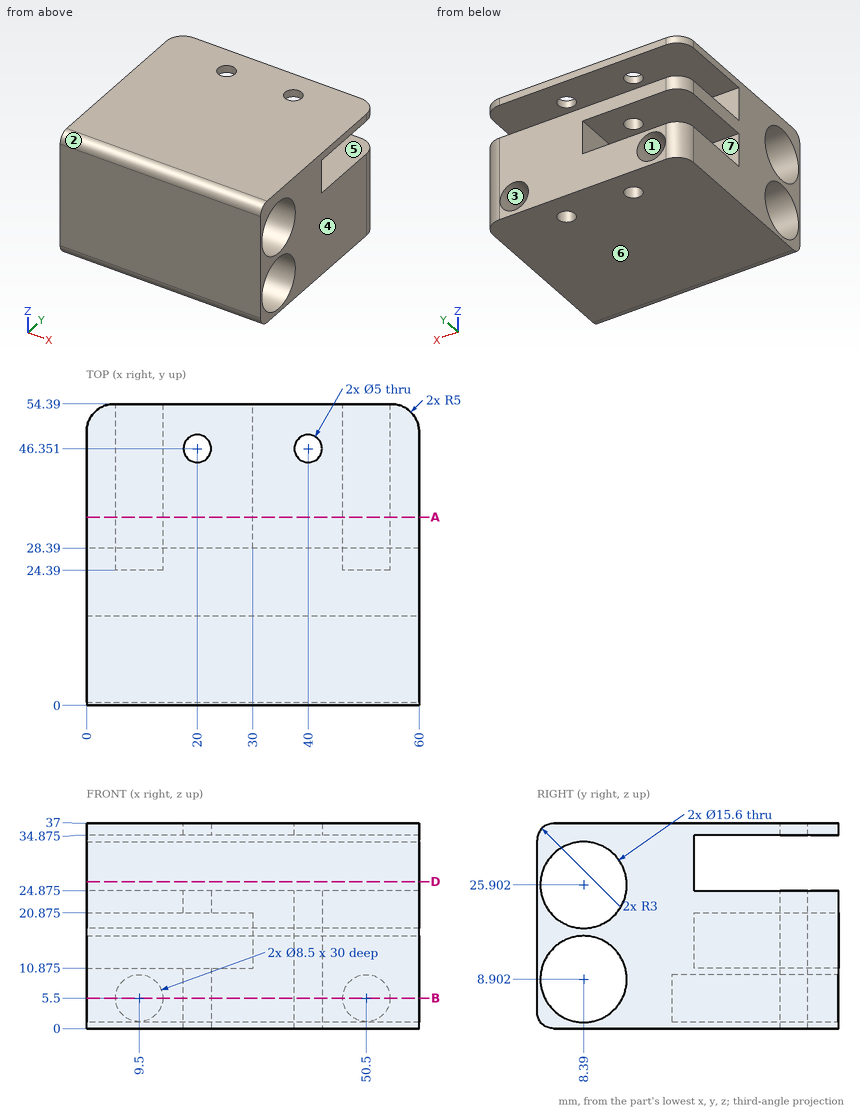
Source: three-view drawing plus pictorial views. Frame: mm from the lowest corner of the part. A direction names the side the tool comes from. Give positions to 0.01 mm unless a question says otherwise; leave off trailing zeros. Order: outer loops, then holes, each group sorted by start corner. A loop starts at its lowest first (then second) coordinate and runs counter-clockwise, first axis right, second up. Notation, with made-up numbers: (-5.75, 69.5) -> (53.25, 69.5) arc R22 cw to (53.25, 90.5) -> close; hole circle Ø1 at (81.25, -34). An arc over 180 degrees is marked (long way). Put each result on its own line as item: value.
Q1. Section D-D, the plane z = 26.5. Return loops of the section in (x, y), then the cut area to 3 significant figures.
Here are the results:
outline: (0, 0) -> (60, 0) -> (60, 0.61) -> (0, 0.61) -> close; (0, 16.17) -> (60, 16.17) -> (60, 28.39) -> (0, 28.39) -> close
area: 770 mm^2
Q2. Material intervals for L1, parallel to Z at x = 25, y = 34.5 (1 decimal); L2, parallel to X at y = 48, z = 3.5; L3, parallel to Z at x = 9, y = 46 (1 decimal), sorted ascending.
Here are the results:
L1: z = 0 to 10.9, 20.9 to 24.9, 34.9 to 37
L2: x = 0 to 5.75, 13.25 to 18.12, 21.88 to 38.12, 41.88 to 46.75, 54.25 to 60
L3: z = 0 to 1.3, 9.7 to 10.9, 20.9 to 24.9, 34.9 to 37
Q3. Section B-B, the plane z = 5.5. Return loops of the section in (x, y).
Here are the results:
outline: (0, 0) -> (60, 0) -> (60, 1.37) -> (0, 1.37) -> close; (0, 15.41) -> (60, 15.41) -> (60, 49.39) arc R5 ccw to (55, 54.39) -> (54.75, 54.39) -> (54.75, 24.39) -> (46.25, 24.39) -> (46.25, 54.39) -> (13.75, 54.39) -> (13.75, 24.39) -> (5.25, 24.39) -> (5.25, 54.39) -> (5, 54.39) arc R5 ccw to (0, 49.39) -> close; hole circle Ø5 at (20, 46.35); hole circle Ø5 at (40, 46.35)
Q4. Reachability of the marked faces 5, 6 and 7 from +Z, -Z, +X, -X, +Y, -Y: full face, straight path, thin tool, end or side. Return the list, or none.
Here are the results:
face 5: +X, -X, +Y
face 6: -Z, +X, -X, +Y, -Y
face 7: -X, +Y
Q5. Section A-A, the plane y = 34. Count the separate pieces of the cut face and the enclosed holes in it, then the cut area to 3 significant figures.
Here are the results:
separate pieces: 2
enclosed holes: 2
area: 1,210 mm^2
Q6. Pin query (flat end, axial travel): pin 1 (1 mm diameter, centred on x = 11, z = 13.5, fed in from +Y); pin 2 (6.5 mm diameter, centred on x = 20, y = 46.35, fed in from -Z); pin 3 (5 mm diameter, centred on y = 40, z = 15.5, fed in from -X); pin 4 (14 mm diameter, centred on y = 8.39, z = 8.9, fed in from -X). Return the tip coordinate at first contact, or that it passes through.
Here are the results:
pin 1: stops at y = 28.39
pin 2: stops at z = 0
pin 3: stops at x = 30
pin 4: passes through
Q7. Draft query along X for the marked faces 1, 2, 3 and 4. Return one class per face: released by +X, released by -X, zero draft, split by the parting line, or undercut.
Here are the results:
face 1: undercut
face 2: zero draft
face 3: undercut
face 4: released by +X
